Autodesk Inventor part; units mm, degrees
ref_plane "YZ Plane" through (0, 0, 0) normal (1, 0, 0) x (0, 1, 0)
ref_plane "XZ Plane" through (0, 0, 0) normal (0, 1, 0) x (-1, 0, 0)
ref_plane "XY Plane" through (0, 0, 0) normal (0, 0, 1) x (1, 0, 0)
sketch "Sketch1" plane through (0, 0, 0) normal (0, 0, 1) x (1, 0, 0)
  line L0 (13.5, -2.5) -> (13.5, 0)
  line L1 (12, 0) -> (13.5, 0)
  line L2 (12, 0) -> (12, -2)
  arc A0 (8, -2) -> (12, -2) centre (10, -2) ccw
  line L3 (8, -2) -> (8, 0)
  line L4 (6.5, 0) -> (8, 0)
  line L5 (6.5, 0) -> (6.5, -2.5)
  line L6 (6.5, -2.5) -> (4, -2.5)
  line L7 (4, -2.5) -> (4, 0)
  line L8 (0, 0) -> (4, 0)
  line L9 (0, 0) -> (0, -8)
  line L10 (20, -8) -> (0, -8)
  line L11 (20, 0) -> (20, -8)
  line L12 (16, 0) -> (20, 0)
  line L13 (16, 0) -> (16, -2.5)
  line L14 (16, -2.5) -> (13.5, -2.5)
  circle A1 centre (5.25, -1.25) radius 1.25
  circle A2 centre (14.75, -1.25) radius 1.25
  line L15 (20, 1) -> (20, -9)
  line L16 (20, -9) -> (0, -9)
  line L17 (0, -9) -> (0, 1)
  line L18 (0, 1) -> (20, 1)
  line L19 (17.25, 1) -> (16.25, 2)
  line L20 (13.25, 2) -> (12.25, 1)
  line L21 (7.75, 1) -> (6.75, 2)
  line L22 (2.75, 1) -> (3.75, 2)
  line L23 (3.75, 2) -> (6.75, 2)
  line L24 (13.25, 2) -> (16.25, 2)
  dimension "d0" = 9
  dimension "d3" = 45
  dimension "d4" = 45
  dimension "d5" = 45
  dimension "d6" = 3
  dimension "d7" = 3
  dimension "d8" = 1.5
  dimension "d9" = 2.5
  dimension "d10" = 2.5
  dimension "d11" = 1.5
extrude "Extrusion1" add sketch "Sketch1" along normal blind 6.4 contours L14 L13 L12 L11 L10 L9 L8 L7 L6 L5 L4 L3 A0 L2 L1 L0 | L0 A2 L14 | L0 L1 L2 A0 L3 L4 L5 A1 L7 L8 L17 L18 L15 L12 L13 A2 | A2 L13 L14 | L15 L16 L17 L10 | L18 L20 L24 L19 | L5 L6 A1 | L18 L22 L23 L21 | A1 L6 L7
sketch "Sketch2" plane through (0, 0, 6.4) normal (0, 0, 1) x (1, 0, 0)
  line L0 (0, -9) -> (20, -9)
  line L1 (20, 1) -> (17.25, 1)
  line L2 (16.5219, -9) -> (16.5219, -9.7169)
  line L3 (16.5219, -9.7169) -> (1, -13)
  line L4 (1, -13) -> (1.0938, -13.4435)
  line L5 (1.0938, -13.4435) -> (17, -9.8474)
  line L6 (17, -9.8474) -> (17, -9)
  point P0 (0, 0)
extrude "Extrusion2" add sketch "Sketch2" against normal blind 6.4
properties material "ABS Plastic"
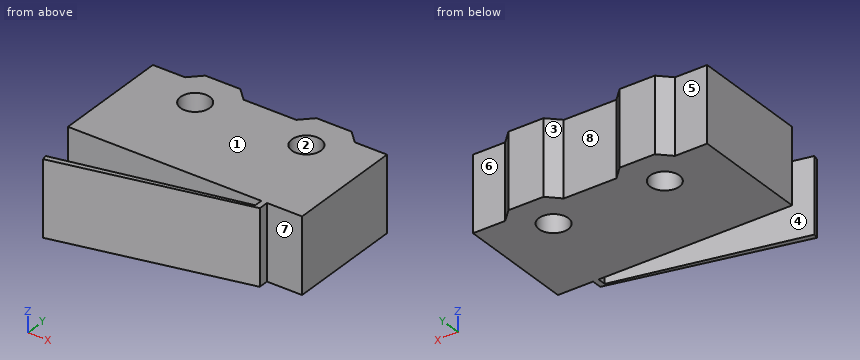
The listing builds one solid part. Answer for the finished solid, in the listing's coordinates (mm). Face numbers are marked on the shaded views. A direction names the side the tool comes from. Coordinates: 2 decimals unless noted, no trailing zeros. Write each loop counter-clockwise with the first axis right and the second up, starting at its lowest first coordinate (ties: lowest second). Pieces come first, ordered by that corner, then holes. Notation, with made-up numbers: (4.25, -24) -> (35.25, -24) arc R20 ccw to (35.25, -19) -> close; hole circle Ø3 at (-13, -14). An arc over 180 degrees is marked (long way). Write each question's results on one line, items separated by ' | '. Start each with the question number.
1) A cutting plane is placed at B-B (z = 4.75). Determine the outline of the cut face in (x, y).
2) A cutting plane is placed at C-C (x = 14). Determine the outline of the cut face in (y, z), then the cut area to 3 significant figures.
3) A cutting plane is placed at D-D (x = 2). Determine the outline of the cut face in (y, z).
4) A tool of negligible diameter and unlimited length cuts with its end or side. For the marked faces 4, 5, 6, 7 and 8, from which of +Z, -Z, +X, -X, +Y, -Y can it reach the whole face along a straight path? Write none if from no direction.
5) Flat-ended cylindrical pins translate along their axes: pin 1 Ø0.8 at (x, z) = (1.5, 2.5) entering from +Y; pin 2 Ø1.5 at (x, y) = (14.75, -1.25) entering from +Z; pin 3 Ø3 at (x, y) = (5.25, -1.25) entering from +Z; pin 4 Ø3.5 at (x, z) = (18, 2) entering from -Y. Find the tip coordinate at first contact, or state that the pin passes through.
6) A cutting plane is placed at A-A (y = -1.25). Determine the outline of the cut face in (x, z), then the cut area to 3 significant figures.
7) Straight lines are drawn through the part: probe 1 along X at (y, z) = (-1.25, 2.25); probe 2 along Y at (x, z) = (5.25, 3.5); probe 3 along Y at (x, z) = (5, 1). For each, find the intervals that lie inside material, in ascending order.
8) For a pull along Y with two mould halves and no side action, classify the marked faces 1, 2 and 3 as +Y half, -Y half, draft (parallel to the pull), parting line (faces both ways), or undercut.
Values follow:
1) outline: (0, -9) -> (16.52, -9) -> (16.52, -9.72) -> (1, -13) -> (1.09, -13.44) -> (17, -9.85) -> (17, -9) -> (20, -9) -> (20, 1) -> (17.25, 1) -> (16.25, 2) -> (13.25, 2) -> (12.25, 1) -> (7.75, 1) -> (6.75, 2) -> (3.75, 2) -> (2.75, 1) -> (0, 1) -> close; hole circle Ø2.5 at (5.25, -1.25); hole circle Ø2.5 at (14.75, -1.25)
2) outline: (-10.53, 0) -> (-10.25, 0) -> (-10.25, 6.4) -> (-10.53, 6.4) -> close; (-9, 0) -> (-2.25, 0) -> (-2.25, 6.4) -> (-9, 6.4) -> close; (-0.25, 0) -> (2, 0) -> (2, 6.4) -> (-0.25, 6.4) -> close | area: 59.4 mm²
3) outline: (-13.24, 0) -> (-12.79, 0) -> (-12.79, 6.4) -> (-13.24, 6.4) -> close; (-9, 0) -> (1, 0) -> (1, 6.4) -> (-9, 6.4) -> close
4) face 4: +Z, -Z, -X | face 5: +Z, -Z, -X, +Y | face 6: +Z, -Z, +X, +Y | face 7: +Z, -Z, +X, -Y | face 8: +Z, -Z, +Y
5) pin 1: y = 1 | pin 2: through | pin 3: z = 6.4 | pin 4: y = -10.02
6) outline: (0, 0) -> (4, 0) -> (4, 6.4) -> (0, 6.4) -> close; (6.5, 0) -> (13.5, 0) -> (13.5, 6.4) -> (6.5, 6.4) -> close; (16, 0) -> (20, 0) -> (20, 6.4) -> (16, 6.4) -> close | area: 96.0 mm²
7) probe 1: 0 to 4, 6.5 to 13.5, 16 to 20 | probe 2: -12.5 to -12.1, -9 to -2.5, 0 to 2 | probe 3: -12.56 to -12.15, -9 to -2.47, -0.03 to 2
8) face 1: draft | face 2: undercut | face 3: +Y half
